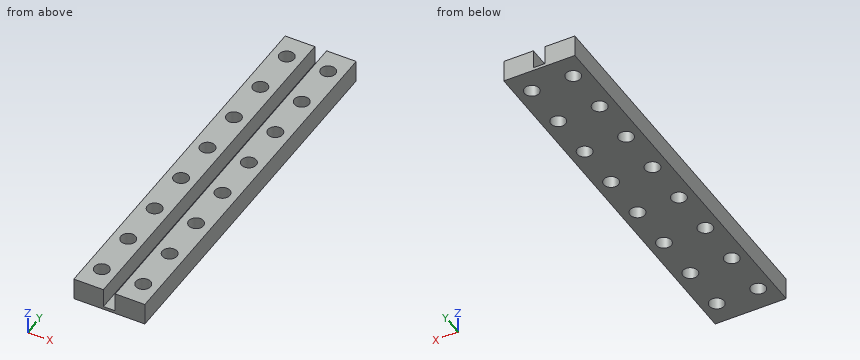
from build123d import *

# Parameters (mm, degrees)
BASE_DEPTH  = 128
ESQUISSE2_R = 2.5
TROU_DEPTH  = 129.779850908


with BuildPart() as part:
    # Esquisse1 → BASE (new body)
    with BuildSketch(Plane(origin=(0, 0, 0), x_dir=(1, 0, 0), z_dir=(0, 1, 0))):
        Polygon((-2, -3.75), (-2, 2.75), (2, 2.75), (2, -3.75), (12, -3.75), (12, 3.75), (-12, 3.75), (-12, -3.75), align=None)
    extrude(amount=-BASE_DEPTH)

    # Esquisse2 → TROU (cut, through all)
    with BuildSketch(Plane.XY.offset(3.75)):
        with Locations((-7, -8)):
            Circle(ESQUISSE2_R)
        with Locations((7, -8)):
            Circle(ESQUISSE2_R)
        with Locations((7, -24)):
            Circle(ESQUISSE2_R)
        with Locations((7, -40)):
            Circle(ESQUISSE2_R)
        with Locations((7, -56)):
            Circle(ESQUISSE2_R)
        with Locations((7, -72)):
            Circle(ESQUISSE2_R)
        with Locations((7, -88)):
            Circle(ESQUISSE2_R)
        with Locations((7, -104)):
            Circle(ESQUISSE2_R)
        with Locations((7, -120)):
            Circle(ESQUISSE2_R)
        with Locations((-7, -24)):
            Circle(ESQUISSE2_R)
        with Locations((-7, -40)):
            Circle(ESQUISSE2_R)
        with Locations((-7, -56)):
            Circle(ESQUISSE2_R)
        with Locations((-7, -72)):
            Circle(ESQUISSE2_R)
        with Locations((-7, -88)):
            Circle(ESQUISSE2_R)
        with Locations((-7, -104)):
            Circle(ESQUISSE2_R)
        with Locations((-7, -120)):
            Circle(ESQUISSE2_R)
    extrude(amount=-TROU_DEPTH, mode=Mode.SUBTRACT)


solid = part.part
Design review of the part built by this model. Coordinates are the model's own, in mm. Round coordinates to 2 decimals unless told otherwise and drop trailing zeros. Write each loop counter-clockwise with the first axis right and the second up, starting at its lowest first coordinate (ties: lowest second). Pieces come first, ordered by that corner, then holes. Notation, with made-up numbers: (30.25, -19) - (43.25, -19) arc R22 cw to (43.25, 13) - close; hole circle Ø11 at (68.25, 22.25). An arc over 180 degrees is marked (long way). Return JSON: item names as keys, results as strings. Group by question number.
Item 1: We need section A-A on z = -0.5. Give the number of separate pieces and of enclosed holes in the cut face, and give its area (3 significant figures).
Item 2: We need section D-D on y = -16. Write out the cut boundary in (x, z), and give its area (3 significant figures).
Item 3: We need section B-B on y = -72. Write out the cut boundary in (x, z), and give its area (3 significant figures).
Item 4: Insertion check: P1, Ø4.5, axis at x = -7, y = -24, coming from the +Z side; P2, Ø6.5, axis at x = 7, y = -24, coming from the -Z side. Each pin has a flat end and moves straight along its axis. Give the tip position at first contact, or say it passes through.
Item 5: For probe 1 along X at (y, z) = (-112.5, 0.25); probe 2 along X at (y, z) = (-42, -0.75); probe 3 along X at (y, z) = (-25, -1), list the stretches that pass through material, from the lowest coordinate up. Write a range as [from, to].
Model answer:
{
 "1": {"separate pieces": "2", "enclosed holes": "16", "area": "2,250 mm²"},
 "2": {"outline": "(-12, -3.75) - (12, -3.75) - (12, 3.75) - (2, 3.75) - (2, -2.75) - (-2, -2.75) - (-2, 3.75) - (-12, 3.75) - close", "area": "154 mm²"},
 "3": {"outline": "(-12, -3.75) - (-9.5, -3.75) - (-9.5, 3.75) - (-12, 3.75) - close; (-4.5, -3.75) - (4.5, -3.75) - (4.5, 3.75) - (2, 3.75) - (2, -2.75) - (-2, -2.75) - (-2, 3.75) - (-4.5, 3.75) - close; (9.5, -3.75) - (12, -3.75) - (12, 3.75) - (9.5, 3.75) - close", "area": "79.0 mm²"},
 "4": {"P1": "passes through", "P2": "stops at z = -3.75"},
 "5": {"probe 1": "x = [-12, -2], [2, 12]", "probe 2": "x = [-12, -8.5], [-5.5, -2], [2, 5.5], [8.5, 12]", "probe 3": "x = [-12, -9.29], [-4.71, -2], [2, 4.71], [9.29, 12]"}
}
